```python
from build123d import *

# Parameters (mm, degrees)
SKETCH1_R           = 3.2639
SKETCH1_R_2         = 2.5019
SKETCH1_R_3         = 6.985
SKETCH1_R_4         = 2.159
SKETCH1_R_5         = 19.05
SKETCH1_R_6         = 4.7625
BOSS_EXTRUDE1_DEPTH = 1.4478


with BuildPart() as part:
    # Sketch1 → Boss-Extrude1 (new body)
    with BuildSketch(Plane(origin=(0, 0, 0), x_dir=(1, 0, 0), z_dir=(0, 1, 0))):
        with BuildLine():
            Line((-70.748540962, -286.823205678), (-108.848540962, -286.823205678))
            ThreePointArc((-108.848540962, -286.823205678), (-126.809053204, -279.38371792), (-134.248540962, -261.423205678))
            Line((-134.248540962, -261.423205678), (-134.248540962, -223.323205678))
            ThreePointArc((-134.248540962, -223.323205678), (-130.528797083, -214.342949557), (-121.548540962, -210.623205678))
            Line((-121.548540962, -210.623205678), (208.651459038, -210.623205678))
            ThreePointArc((208.651459038, -210.623205678), (217.631715159, -214.342949557), (221.351459038, -223.323205678))
            Line((221.351459038, -223.323205678), (221.351459038, -261.423205678))
            ThreePointArc((221.351459038, -261.423205678), (213.911971281, -279.38371792), (195.951459038, -286.823205678))
            Line((195.951459038, -286.823205678), (157.851459038, -286.823205678))
            Line((157.851459038, -286.823205678), (157.851459038, -328.098205678))
            ThreePointArc((157.851459038, -328.098205678), (155.991587099, -332.588333738), (151.501459038, -334.448205678))
            Line((151.501459038, -334.448205678), (-64.398540962, -334.448205678))
            ThreePointArc((-64.398540962, -334.448205678), (-68.888669022, -332.588333738), (-70.748540962, -328.098205678))
            Line((-70.748540962, -328.098205678), (-70.748540962, -286.823205678))
        make_face()
        with Locations(Location((27.676459038, -291.649205678, 0), (0, 0, 270))):
            Circle(SKETCH1_R, mode=Mode.SUBTRACT)
        with Locations(Location((43.551459038, -291.649205678, 0), (0, 0, 270))):
            Circle(SKETCH1_R, mode=Mode.SUBTRACT)
        with Locations(Location((59.426459038, -291.649205678, 0), (0, 0, 270))):
            Circle(SKETCH1_R, mode=Mode.SUBTRACT)
        with Locations(Location((-28.025740962, -215.246005678, 0), (0, 0, 270))):
            Circle(SKETCH1_R_2, mode=Mode.SUBTRACT)
        with Locations(Location((-28.025740962, -262.388405678, 0), (0, 0, 90))):
            Circle(SKETCH1_R_2, mode=Mode.SUBTRACT)
        with Locations(Location((19.116659038, -215.246005678, 0), (0, 0, 90))):
            Circle(SKETCH1_R_2, mode=Mode.SUBTRACT)
        with Locations(Location((19.116659038, -262.388405678, 0), (0, 0, 270))):
            Circle(SKETCH1_R_2, mode=Mode.SUBTRACT)
        with Locations(Location((27.676459038, -313.874205678, 0), (0, 0, 270))):
            Circle(SKETCH1_R, mode=Mode.SUBTRACT)
        with Locations(Location((43.551459038, -313.874205678, 0), (0, 0, 270))):
            Circle(SKETCH1_R, mode=Mode.SUBTRACT)
        with Locations(Location((59.426459038, -313.874205678, 0), (0, 0, 270))):
            Circle(SKETCH1_R, mode=Mode.SUBTRACT)
        with Locations(Location((-58.048540962, -223.323205678, 0), (0, 0, 270))):
            Circle(SKETCH1_R_3, mode=Mode.SUBTRACT)
        with Locations(Location((-67.573540962, -213.798205678, 0), (0, 0, 270))):
            Circle(SKETCH1_R_4, mode=Mode.SUBTRACT)
        with Locations(Location((-48.523540962, -232.848205678, 0), (0, 0, 270))):
            Circle(SKETCH1_R_4, mode=Mode.SUBTRACT)
        with Locations(Location((-4.454540962, -238.817205678, 0), (0, 0, 270))):
            Circle(SKETCH1_R_5, mode=Mode.SUBTRACT)
        with Locations(Location((135.626459038, -232.848205678, 0), (0, 0, 90))):
            Circle(SKETCH1_R_4, mode=Mode.SUBTRACT)
        with Locations(Location((145.151459038, -223.323205678, 0), (0, 0, 90))):
            Circle(SKETCH1_R_3, mode=Mode.SUBTRACT)
        with Locations(Location((154.676459038, -213.798205678, 0), (0, 0, 90))):
            Circle(SKETCH1_R_4, mode=Mode.SUBTRACT)
        with Locations(Location((-121.548540962, -223.323205678, 0), (0, 0, 270))):
            Circle(SKETCH1_R_6, mode=Mode.SUBTRACT)
        with Locations(Location((208.651459038, -223.323205678, 0), (0, 0, 270))):
            Circle(SKETCH1_R_6, mode=Mode.SUBTRACT)
        Polygon((-1.724040962, -304.36377724), (-1.724040962, -297.984634115), (-7.248540962, -294.795062553), (-12.773040962, -297.984634115), (-12.773040962, -304.36377724), (-7.248540962, -307.553348802), align=None, mode=Mode.SUBTRACT)
        Polygon((94.351459038, -307.553348802), (88.826959038, -304.36377724), (88.826959038, -297.984634115), (94.351459038, -294.795062553), (99.875959038, -297.984634115), (99.875959038, -304.36377724), align=None, mode=Mode.SUBTRACT)
        Polygon((-103.324040962, -258.233634115), (-108.848540962, -255.044062553), (-114.373040962, -258.233634115), (-114.373040962, -264.61277724), (-108.848540962, -267.802348802), (-103.324040962, -264.61277724), align=None, mode=Mode.SUBTRACT)
        Polygon((201.475959038, -264.61277724), (195.951459038, -267.802348802), (190.426959038, -264.61277724), (190.426959038, -258.233634115), (195.951459038, -255.044062553), (201.475959038, -258.233634115), align=None, mode=Mode.SUBTRACT)
    extrude(amount=BOSS_EXTRUDE1_DEPTH)


solid = part.part
```
Can you work these out from the model? Positions are in its coordinate system, mm. Give positions to 0.01 mm unless a question says otherwise; leave off trailing zeros. Loops run counter-clockwise (first coordinate to the right, second up) from the corner with the lowest first, then second, coordinate; pieces in that order, holes last. Notation, with made-up numbers: M 7,31.25 L 36,31.25 A20 cw 36,60.25 Z; hole C 54,25.25 d2. An arc over 180 degrees is marked long. Answer in a Markdown table with one row per item.
1. Suppose I cut it at C-C on z = 282. Write out the boundary of the cut face in (x, y), plus the area to 3 significant figures.
Taken from the geometry:
| item | result |
|---|---|
| outline | M -123.74,0 L 210.84,0 L 210.84,1.45 L -123.74,1.45 Z |
| area | 484 mm² |
2. Suppose I cut it at B-B on y = 0.4. Count the separate pieces of the cut face and the enclosed holes in it, plus the area to 3 significant figures.
Taken from the geometry:
| item | result |
|---|---|
| separate pieces | 1 |
| enclosed holes | 23 |
| area | 35,300 mm² |
3. Suppose I cut it at A-A on z = 249. Write out the boundary of the cut face in (x, y), plus the area to 3 significant figures.
Taken from the geometry:
| item | result |
|---|---|
| outline | M -134.25,0 L -20.55,0 L -20.55,1.45 L -134.25,1.45 Z; M 11.65,0 L 221.35,0 L 221.35,1.45 L 11.65,1.45 Z |
| area | 468 mm² |
4. If I drill on line 1 along X through (y, z) = (0.5, 299.5); line 2 along X through (y, z) = (0.2, 314.5); line 3 along Z through (x, y) = (-6, 0.2), over which ranges is the centre line in solid material (lowest first)?
Taken from the geometry:
| item | result |
|---|---|
| line 1 | x = -70.75 to -12.77, -1.72 to 88.83, 99.88 to 157.85 |
| line 2 | x = -70.75 to 24.47, 30.88 to 40.35, 46.75 to 56.22, 62.63 to 157.85 |
| line 3 | z = 210.62 to 219.83, 257.8 to 295.52, 306.83 to 334.45 |
5. For pin 1 Ø0.7 at (y, z) = (0.5, 262.5) entering from -X; pin 2 Ø4.5 at (x, z) = (19.12, 215.25) entering from +Y, each with a flat end and sliding along its axis, tell me the tip position at first contact or that it passes through.
Taken from the geometry:
| item | result |
|---|---|
| pin 1 | stops at x = -134.24 |
| pin 2 | passes through |
6. Thinking about a two-plate mould opening in X: for faces 1 (the cylindrical face through (217.53, 0.71, 214.24)), 2 (the cylindrical face through (-3.617, 0.714, 219.786)), 3 (the flat face through (46, 1.448, 258)), which applies, released by +X, released by -X, zero draft, split by the parting line, or undercut?
Taken from the geometry:
| item | result |
|---|---|
| face 1 | released by +X |
| face 2 | undercut |
| face 3 | zero draft |
